```python
from build123d import *

# Parameters (mm, degrees)
F1_DEPTH = 25
F3_DEPTH = 25


# Not quite as in the source:
# - a feature names something its author has since deleted; it is built from what else it names


with BuildPart() as f1:
    # F0 (on Top) → F1 (new body)
    with BuildSketch(Plane.XY):
        with BuildLine():
            Line((-3, -126.7858377695), (-3, -124.4612824492))
            ThreePointArc((-3, -124.4612824492), (-3.7416573868, -136.7019175526), (7, -130.7858377695))
            ThreePointArc((7, -130.7858377695), (5.9160797831, -127.0441803827), (3, -124.4612824492))
            Line((3, -124.4612824492), (3, -126.7858377695))
            ThreePointArc((3, -126.7858377695), (4.472135955, -128.549769792), (5, -130.7858377695))
            ThreePointArc((5, -130.7858377695), (-2.2360679775, -135.2579737245), (-3, -126.7858377695))
        make_face()
        with BuildLine():
            ThreePointArc((3, -9.5393920142), (0, -10), (-3, -9.5393920142))
            Line((-3, -9.5393920142), (-3, -124.4612824492))
            ThreePointArc((-3, -124.4612824492), (0, -123.7858377695), (3, -124.4612824492))
            Line((3, -124.4612824492), (3, -9.5393920142))
        make_face()
        with BuildLine():
            ThreePointArc((3, -124.4612824492), (0, -123.7858377695), (-3, -124.4612824492))
            Line((-3, -124.4612824492), (-3, -126.7858377695))
            ThreePointArc((-3, -126.7858377695), (0, -125.7858377695), (3, -126.7858377695))
            Line((3, -126.7858377695), (3, -124.4612824492))
        make_face()
        with BuildLine():
            ThreePointArc((-3, -2.6457513111), (-1.4142135624, 3.7416573868), (4, 0))
            ThreePointArc((4, 0), (3.7416573868, -1.4142135624), (3, -2.6457513111))
            Line((3, -2.6457513111), (3, -9.5393920142))
            ThreePointArc((3, -9.5393920142), (8.0622577483, -5.9160797831), (10, 0))
            ThreePointArc((10, 0), (-5.9160797831, 8.0622577483), (-3, -9.5393920142))
            Line((-3, -9.5393920142), (-3, -2.6457513111))
        make_face()
        with BuildLine():
            ThreePointArc((3, -2.6457513111), (0, -4), (-3, -2.6457513111))
            Line((-3, -2.6457513111), (-3, -9.5393920142))
            ThreePointArc((-3, -9.5393920142), (0, -10), (3, -9.5393920142))
            Line((3, -9.5393920142), (3, -2.6457513111))
        make_face()
    extrude(amount=F1_DEPTH)

    # F2 (on Top) → F3 (join)
    with BuildSketch(Plane.XY):
        with BuildLine():
            Line((35, 0), (4, 0))
            ThreePointArc((4, 0), (0, -4), (-4, 0))
            Line((-4, 0), (-35, 0))
            Line((-35, 0), (-35, -6))
            Line((-35, -6), (35, -6))
            Line((35, -6), (35, 0))
        make_face()
    extrude(amount=F3_DEPTH)


solid = f1.part
```
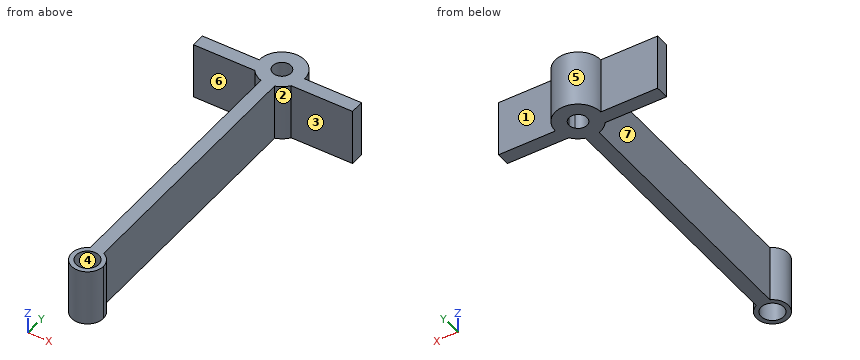
CAD build for the part. Positions are in the model's coordinates, mm. Face numbers are marked on the shaded views. A direction names the side the tool comes from. Round coordinates to 2 decimals unless told otherwise and drop trailing zeros. Write each loop counter-clockwise with the first axis right and the second up, starting at its lowest first coordinate (ties: lowest second). Pieces come first, ordered by that corner, then holes. Notation, with made-up numbers: (31.25, -18) - (80.25, -18) arc R26 cw to (80.25, 10) - close; hole circle Ø2 at (42.5, -26). An arc over 180 degrees is marked (long way). Return JSON: item names as keys, results as strings. Group by question number.
Item 1: Probe probe 1 along Y at (x, z) = (0, 12.5); probe 2 along Y at (x, z) = (-26, 18.5); probe 3 along Y at (x, z) = (5.5, 8). List the from-to ranges inside material, lowest first.
Item 2: Band-saw the part on A-A on x = 0. List the corners of the cut face in (y, z), plus the area to 3 significant figures.
Item 3: 3-axis set-ups, long thin cutter, end or side, ignore diameter. For the marked faces 1, 2 and 3: which of +Z, -Z, +X, -X, +Y, -Y reach the whole face in a straight line?
Item 4: Band-saw the part on C-C on x = 12. List the corners of the cut face in (y, z), plus the area to 3 significant figures.
Item 5: Flat gauge pins, fed straight in: pin 1 Ø4 at (x, z) = (19.5, 19.5) entering from -Y; pin 2 Ø7.5 at (x, z) = (17, 14.5) entering from +Y; pin 3 Ø5 at (y, z) = (-120.5, 18.5) entering from +X; pin 4 Ø10.5 at (x, y) = (0, 0) entering from +Z. Where does each tip first touch, or does it go through?
Item 6: Mould opens along Y. For the marked faces 4, 5, 6 and 7 say: +Y half, -Y half, draft (parallel to the pull), parting line (faces both ways), or undercut.
Item 7: Band-saw the part on D-D on y = -32. List the corners of the cut face in (x, z).
Item 8: Band-saw the part on B-B on z = 3. List the corners of the cut face in (x, y).
Resolved:
{
 "1": {"probe 1": "y = -137.79 to -135.79, -125.79 to -4, 4 to 10", "probe 2": "y = -6 to 0", "probe 3": "y = -135.12 to -126.46, -8.35 to 8.35"},
 "2": {"outline": "(-137.79, 0) - (-135.79, 0) - (-135.79, 25) - (-137.79, 25) - close; (-125.79, 0) - (-4, 0) - (-4, 25) - (-125.79, 25) - close; (4, 0) - (10, 0) - (10, 25) - (4, 25) - close", "area": "3,240 mm²"},
 "3": {"face 1": "+Z, -Z, +X, +Y", "face 2": "+Z, -Z, +X", "face 3": "+Z, -Z, +X, -Y"},
 "4": {"outline": "(-6, 0) - (0, 0) - (0, 25) - (-6, 25) - close", "area": "150 mm²"},
 "5": {"pin 1": "stops at y = -6", "pin 2": "stops at y = 0", "pin 3": "stops at x = 3", "pin 4": "stops at z = 25"},
 "6": {"face 4": "undercut", "face 5": "+Y half", "face 6": "-Y half", "face 7": "undercut"},
 "7": {"outline": "(-3, 0) - (3, 0) - (3, 25) - (-3, 25) - close"},
 "8": {"outline": "(-35, -6) - (-8, -6) arc R10 ccw to (-3, -9.54) - (-3, -124.46) arc R7 ccw (long way) to (3, -124.46) - (3, -9.54) arc R10 ccw to (8, -6) - (35, -6) - (35, 0) - (10, 0) arc R10 ccw to (-10, 0) - (-35, 0) - close; hole circle Ø10 at (0, -130.79); hole circle Ø8 at (0, 0)"}
}
